Part model, mm, in its own coordinate system. A direction names the side the tool comes from. Round coordinates to 2 decimals unless told otherwise and drop trailing zeros. Loops run counter-clockwise (first coordinate to the right, second up) from the corner with the lowest first, then second, coordinate; pieces in that order, holes last. Notation, with made-up numbers: M 62.25,80 L 90.25,80 A30 cw 90.25,106 Z; hole C 18,84.5 d8. An arc over 180 degrees is marked long. Write each question's results on one line, items separated by ' | '.
Autodesk Fusion 360 part; units mm, degrees
sketch "Esquisse1" plane through (0, 0, 0) normal (0, 0, 1) x (1, 0, 0)
  line L0 (-30.5, 8.75) -> (30.5, 8.75)
  line L1 (30.5, 8.75) -> (30.5, -8.75)
  line L2 (30.5, -8.75) -> (-30.5, -8.75)
  line L3 (-30.5, -8.75) -> (-30.5, 8.75)
  line L4 (-32.35, 10.9) -> (32.35, 10.9)
  line L5 (32.35, 10.9) -> (32.35, -10.9)
  line L6 (32.35, -10.9) -> (-32.35, -10.9)
  line L7 (-32.35, -10.9) -> (-32.35, 10.9)
  dimension "d1" = 61
  dimension "d2" = 17.5
  dimension "d3" = 30.5
  dimension "d4" = 8.75
  dimension "d5" = 64.7
  dimension "d6" = 21.8
  dimension "d7" = 32.35
  dimension "d8" = 10.9
extrude "Extrusion1" add sketch "Esquisse1" along normal blind 16 contours L0 L1 L2 L3
extrude "Extrusion2" add sketch "Esquisse1" along normal blind 2
Item 1: Drop flat-ended pins along their axis: P1, Ø4, axis at x = 15, z = 6.5, coming from the +Y side; P2, Ø1, axis at x = -20.5, z = 13, coming from the -Y side; P3, Ø8, axis at y = -6, z = 14, coming from the -X side. Give the stop position or say it passes through.
Filled sheet:
P1: y = 8.75 | P2: y = -8.75 | P3: x = -30.5
Item 2: Which spindle directions (+Z, -Z, +X, -X, +Y, -Y) get a long thin tool onto all of the face, cutting with end or side? Do faces 1 (the flat face through (30.5, 0, 9)), 2 (the flat face through (0, 8.75, 9)), 3 (the flat face through (-30.5, 0, 9)), 4 (the flat face through (0, -8.75, 9)). Say none if no direction does.
Filled sheet:
face 1: +Z, +X, +Y, -Y | face 2: +Z, +X, -X, +Y | face 3: +Z, -X, +Y, -Y | face 4: +Z, +X, -X, -Y
Item 3: Band-saw the part on C-C on z = 6.75. Give the cut face in (x, y), and give its area (3 significant figures).
Filled sheet:
outline: M -30.5,-8.75 L 30.5,-8.75 L 30.5,8.75 L -30.5,8.75 Z | area: 1,070 mm^2
Item 4: Band-saw the part on A-A on y = 4.25. Give the cut face in (x, z).
Filled sheet:
outline: M -32.35,0 L 32.35,0 L 32.35,2 L 30.5,2 L 30.5,16 L -30.5,16 L -30.5,2 L -32.35,2 Z
Item 5: Band-saw the part on B-B on x = 1. Give the cut face in (y, z).
Filled sheet:
outline: M -10.9,0 L 10.9,0 L 10.9,2 L 8.75,2 L 8.75,16 L -8.75,16 L -8.75,2 L -10.9,2 Z
Item 6: Wall check: L1, parallel to X at y = -6.25, z = 9.5; L2, parallel to Y at x = 1, z = 4.5; L3, parallel to Z at x = -28, y = -9.5. Give the ranges that are in metal, low to high.
Filled sheet:
L1: -30.5 to 30.5 | L2: -8.75 to 8.75 | L3: 0 to 2
Item 7: Band-saw the part on D-D on y = -9.5. Give the cut face in (x, z).
Filled sheet:
outline: M -32.35,0 L 32.35,0 L 32.35,2 L -32.35,2 Z
